Source: three-view drawing plus pictorial views. Frame: mm from the lowest corner of the part. A direction names the side the tool comes from. Give positions to 0.01 mm unless a question says otherwise; leave off trailing zeros. Loops run counter-clockwise (first coordinate to the right, second up) from the corner with the lowest first, then second, coordinate; pieces in that order, holes last. Notation, with made-up numbers: (-7, 18.5) - (-3, 18.5) arc R19 cw to (-3, 29.5) - close; hole circle Ø5 at (21, 21). An arc over 180 degrees is marked (long way). Answer as a JSON object with one key per item and string values. Group by question number.
(1) Section query B-B (y = 8). Return loops of the section in (x, z).
(2) Section query C-C (z = 12.5). Return loops of the section in (x, y).
(3) Material intervals for L1, parallel to X at y = 1.45, z = 8; L2, parallel to X at y = 2.2, z = 42; L3, parallel to Z at x = 29, y = 1.3, sorted ascending.
(4) Pin query (flat end, axial travel): P1, Ø4, axis at x = 17.5, z = 37, coming from the +Y side; P2, Ø8, axis at x = 12.5, y = 12, coming from the -Z side; P3, Ø15, axis at x = 25, z = 25, coming from the +Y side. Return the tip coordinate at first contact, or that it passes through.
(5) Section query A-A (y = 1.25). Return loops of the section in (x, z).
(6) Access query for the marked faces 1 and 2. Directions: +Z, -Z, +X, -X, +Y, -Y. A direction counts if a zero-diameter tool reaches every point of the face in a straight line with its end or side. Return the directions, or none.
(7) Section query D-D (x = 17). Return loops of the section in (y, z), plus the area to 3 significant figures.
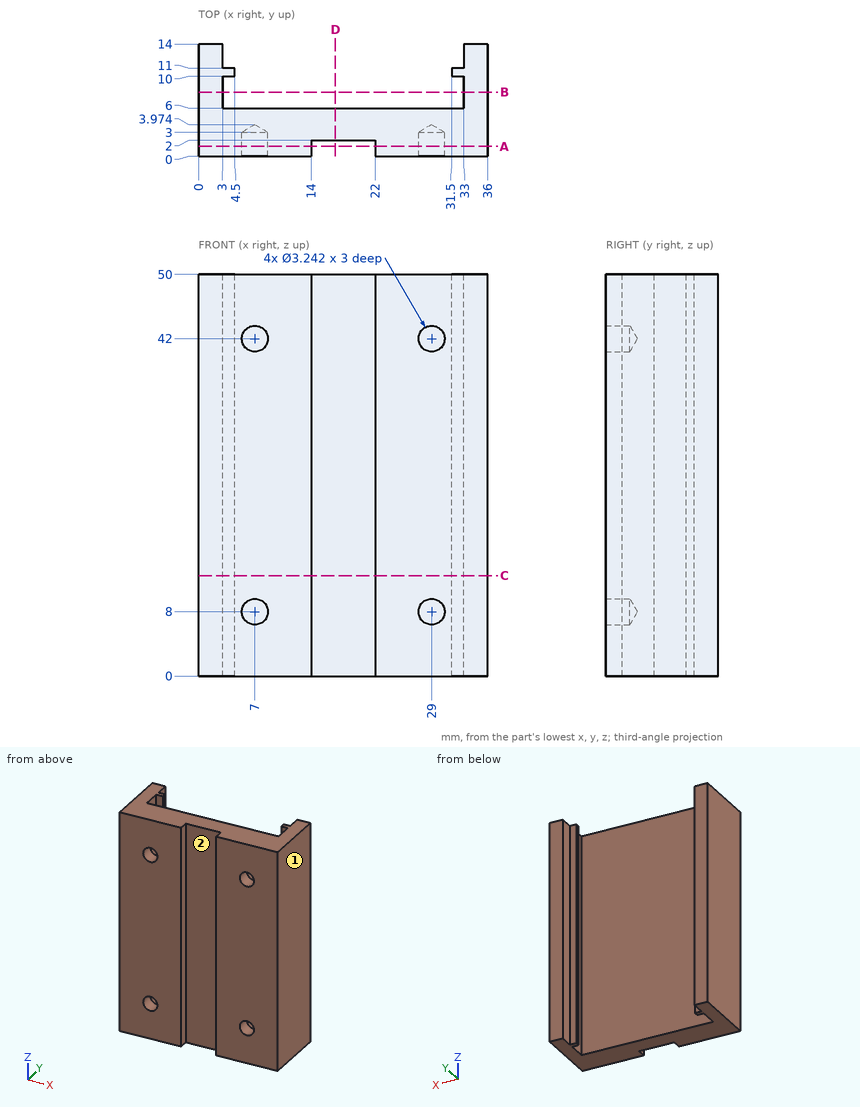
Recorded:
{
 "1": {"outline": "(0, 0) - (3, 0) - (3, 50) - (0, 50) - close; (33, 0) - (36, 0) - (36, 50) - (33, 50) - close"},
 "2": {"outline": "(0, 0) - (14, 0) - (14, 2) - (22, 2) - (22, 0) - (36, 0) - (36, 14) - (33, 14) - (33, 11) - (31.5, 11) - (31.5, 10) - (33, 10) - (33, 6) - (3, 6) - (3, 10) - (4.5, 10) - (4.5, 11) - (3, 11) - (3, 14) - (0, 14) - close"},
 "3": {"L1": "x = 0 to 5.38, 8.62 to 14, 22 to 27.38, 30.62 to 36", "L2": "x = 0 to 5.38, 8.62 to 27.38, 30.62 to 36", "L3": "z = 0 to 6.38, 9.62 to 40.38, 43.62 to 50"},
 "4": {"P1": "stops at y = 6", "P2": "passes through", "P3": "stops at y = 11"},
 "5": {"outline": "(0, 0) - (14, 0) - (14, 50) - (0, 50) - close; (22, 0) - (36, 0) - (36, 50) - (22, 50) - close; hole circle Ø3.24 at (7, 8); hole circle Ø3.24 at (7, 42); hole circle Ø3.24 at (29, 8); hole circle Ø3.24 at (29, 42)"},
 "6": {"face 1": "+Z, -Z, +X, +Y, -Y", "face 2": "+Z, -Z, -Y"},
 "7": {"outline": "(2, 0) - (6, 0) - (6, 50) - (2, 50) - close", "area": "200 mm^2"}
}
